The model under review builds one solid part; all positions refer to its coordinate system, in mm. Face numbers are marked on the shaded views. A direction names the side the tool comes from. Round coordinates to 2 decimals unless told otherwise and drop trailing zeros. Loops run counter-clockwise (first coordinate to the right, second up) from the corner with the lowest first, then second, coordinate; pieces in that order, holes last. Notation, with made-up numbers: M -5.75,-18.5 L 11.25,-18.5 A18 cw 11.25,-3.5 Z; hole C -12,-13.5 d3. An arc over 180 degrees is marked long. Return JSON: item names as keys, results as strings. Group by question number.
Q1. Consider section A-A (x = 0). State the section outline as (y, z) points, and give its area (3 significant figures).
Q2. Clearance check with flat-ended pins moving along their axes: pin 1 Ø5 at (x, z) = (-2, -7) entering from +Y; pin 2 Ø10 at (x, y) = (2, -26.5) entering from -Z. State where each tip first meets the part, or that it passes through.
Q3. Consider section C-C (z = -21.5). State the section outline as (x, y) points.
Q4. For the marked faces 1 and 2, list the 3-axis set-ups (+Z, -Z, +X, -X, +Y, -Y) from which the entire face can be reached by the end or side of a thin tool; tool diameter is ignored.
Q5. Consider section B-B (z = -16.5). State the section outline as (x, y) points, and give its area (3 significant figures).
Q6. Consider section D-D (y = 9). State the section outline as (x, z) points, and give its area (3 significant figures).
Q7. To check wall thickness, follow line 1 along Y through (x, z) = (6.5, -14); line 2 along Z through (x, y) = (7.75, -21); line 3 along Y through (x, z) = (0, 7). State the ranges of each line that lie inside material, in increasing order.
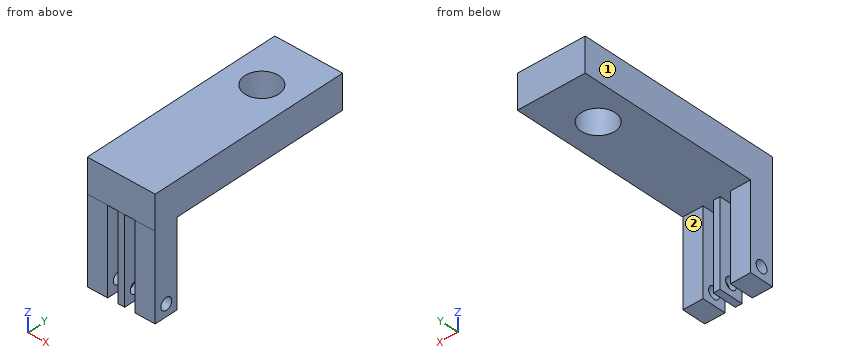
from build123d import *

# Parameters (mm, degrees)
F0_W     = 20
F0_H     = 60
F0_R     = 5
F1_DEPTH = 10
F2_W     = 2
F2_H     = 7.045413
F2_W_2   = 6
F3_DEPTH = 25
F4_R     = 1.75
F5_DEPTH = 25


with BuildPart() as f1:
    # F0 (on Top) → F1 (new body)
    with BuildSketch(Plane.XY):
        with Locations((0, -15.870169)):
            Rectangle(F0_W, F0_H)
        with Locations((0, -0.870169)):
            Circle(F0_R, mode=Mode.SUBTRACT)
    extrude(amount=F1_DEPTH)

    # F2 (on face) → F3 (join)
    with BuildSketch(Plane(origin=(0, 0, 0), x_dir=(1, 0, 0), z_dir=(0, 0, -1))):
        with Locations((0, 42.347462)):
            Rectangle(F2_W, F2_H)
        with Locations((-7, 42.347462)):
            Rectangle(F2_W_2, F2_H)
        with Locations((7, 42.347462)):
            Rectangle(F2_W_2, F2_H)
    extrude(amount=F3_DEPTH)

    # F4 (on face) → F5 (cut)
    with BuildSketch(Plane.YZ.offset(10)):
        with Locations((-42.324756, -21.5)):
            Circle(F4_R)
    extrude(amount=-F5_DEPTH, mode=Mode.SUBTRACT)


solid = f1.part
Values:
{
 "1": {"outline": "M -45.87,-25 L -38.82,-25 L -38.82,0 L -5.87,0 L -5.87,10 L -45.87,10 Z; M 4.13,0 L 14.13,0 L 14.13,10 L 4.13,10 Z; hole C -42.32,-21.5 d3.5", "area": "667 mm2"},
 "2": {"pin 1": "stops at y = -38.82", "pin 2": "stops at z = 0"},
 "3": {"outline": "M -10,-45.87 L -4,-45.87 L -4,-44.07 L -10,-44.07 Z; M -10,-40.57 L -4,-40.57 L -4,-38.82 L -10,-38.82 Z; M -1,-45.87 L 1,-45.87 L 1,-44.07 L -1,-44.07 Z; M -1,-40.57 L 1,-40.57 L 1,-38.82 L -1,-38.82 Z; M 4,-45.87 L 10,-45.87 L 10,-44.07 L 4,-44.07 Z; M 4,-40.57 L 10,-40.57 L 10,-38.82 L 4,-38.82 Z"},
 "4": {"face 1": "+Z, -Z, -X, +Y, -Y", "face 2": "-Z, +X, -X, +Y"},
 "5": {"outline": "M -10,-45.87 L -4,-45.87 L -4,-38.82 L -10,-38.82 Z; M -1,-45.87 L 1,-45.87 L 1,-38.82 L -1,-38.82 Z; M 4,-45.87 L 10,-45.87 L 10,-38.82 L 4,-38.82 Z", "area": "98.6 mm2"},
 "6": {"outline": "M -10,0 L 10,0 L 10,10 L -10,10 Z", "area": "200 mm2"},
 "7": {"line 1": "y = -45.87 to -38.82", "line 2": "z = 0 to 10", "line 3": "y = -45.87 to -5.87, 4.13 to 14.13"}
}
